from build123d import *

# Parameters (mm, degrees)
SKETCH_R        = 4
SKETCH_R_2      = 2.5
PAD_DEPTH       = 25
SKETCH001_W     = 1
SKETCH001_H     = 17.797282
POCKET_DEPTH    = 20
CHAMFER_SIZE    = 0.5
CHAMFER001_SIZE = 0.5


with BuildPart() as part:
    # Sketch → Pad (new body)
    with BuildSketch(Plane.XY):
        Circle(SKETCH_R)
        Circle(SKETCH_R_2, mode=Mode.SUBTRACT)
    extrude(amount=PAD_DEPTH)

    # Sketch001 (on Face4 of Pad) → Pocket (cut)
    with BuildSketch(Plane.XY.offset(25)):
        Rectangle(SKETCH001_W, SKETCH001_H)
    extrude(amount=-POCKET_DEPTH, mode=Mode.SUBTRACT)

    # Chamfer
    chamfer_edges = [part.edges().sort_by_distance(p)[0] for p in [
        (-2.5, 0, 25),
    ]]
    chamfer(chamfer_edges, length=CHAMFER_SIZE)

    # Chamfer001
    chamfer001_edges = [part.edges().sort_by_distance(p)[0] for p in [
        (1.936492, 1.581139, 25),
        (1.936492, -1.581139, 25),
    ]]
    chamfer(chamfer001_edges, length=CHAMFER001_SIZE)


solid = part.part
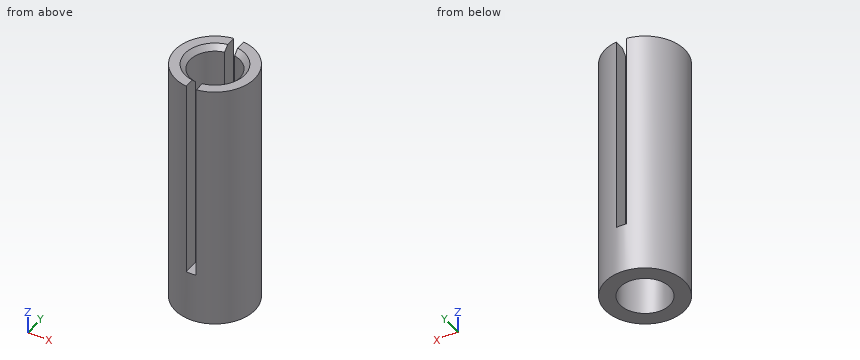
Read the model definition and answer for the solid it produces. Units are mm, in the model's axes. Give positions to 0.01 mm unless a question says otherwise; leave off trailing zeros. Write each loop counter-clockwise with the first axis right and the second up, starting at its lowest first coordinate (ties: lowest second). Pieces come first, ordered by that corner, then holes. Notation, with made-up numbers: (61.5, -25) - (68.5, -25) arc R21 cw to (68.5, -12) - close; hole circle Ø2 at (73.25, -23). An arc over 180 degrees is marked (long way). Answer in a Markdown table with one row per item. Add a question column.
Item 1: Section C-C, the plane z = 16.5 is taken. Write down the section's boundary in (x, y).
Item 2: Section D-D, the plane z = 3.5 is taken. Write down the section's boundary in (x, y), and give its area (3 significant figures).
Item 3: Section B-B, the plane y = 0 is taken. Write down the section's boundary in (x, z).
Item 4: Flat-ended cylindrical pins translate along their axes: P1, Ø0.8, axis at x = 0, y = 3.5, coming from the +Z side; P2, Ø4, axis at x = 0.5, z = 8, coming from the -Y side; P3, Ø0.8, axis at y = 3.5, z = 19.5, coming from the +X side. Find the tip coordinate at first contact, or state that the pin passes through.
Item 5: Find the intervals of material crossed by L1, parallel to X at y = 0, z = 6.25; L2, parallel to X at y = -0.5, z = 12.75; L3, parallel to Y at x = 2.25, z = 17.25, in increasing order.
Item 6: Section A-A, the plane x = 0 is taken. Write down the section's boundary in (y, z), and give its area (3 significant figures).
Recorded:
| question | item | result |
|---|---|---|
| 1 | outline | (-0.5, -3.97) - (-0.5, -2.45) arc R2.5 cw to (-0.5, 2.45) - (-0.5, 3.97) arc R4 ccw to start; (0.5, -3.97) arc R4 ccw to (0.5, 3.97) - (0.5, 2.45) arc R2.5 cw to (0.5, -2.45) - close |
| 2 | outline | circle Ø8 at (0, 0); hole circle Ø5 at (0, 0) |
| 2 | area | 30.6 mm2 |
| 3 | outline | (-4, 0) - (-2.5, 0) - (-2.5, 24.5) - (-3, 25) - (-4, 25) - close; (2.5, 0) - (4, 0) - (4, 25) - (3, 25) - (2.5, 24.5) - close |
| 4 | P1 | stops at z = 5 |
| 4 | P2 | stops at y = -3.97 |
| 4 | P3 | stops at x = 2.53 |
| 5 | L1 | x = -4 to -2.5, 2.5 to 4 |
| 5 | L2 | x = -3.97 to -2.45, 2.45 to 3.97 |
| 5 | L3 | y = -3.31 to -1.09, 1.09 to 3.31 |
| 6 | outline | (-4, 0) - (-2.5, 0) - (-2.5, 5) - (-4, 5) - close; (2.5, 0) - (4, 0) - (4, 5) - (2.5, 5) - close |
| 6 | area | 15.0 mm2 |
